Design review of the part shown in the three views and the two pictorial views. Dimensions are in mm from the part's minimum x, y and z. Coordinates: 2 decimals unless noted, no trailing zeros. Loops run counter-clockwise (first coordinate to the right, second up) from the corner with the lowest first, then second, coordinate; pieces in that order, holes last. Notation, with made-up numbers: (-33, 42) -> (6, 42) arc R21 ccw to (6, 54) -> close; hole circle Ø7 at (68.5, 56.25). An arc over 180 degrees is marked (long way). Answer in a Markdown table with one row per item.
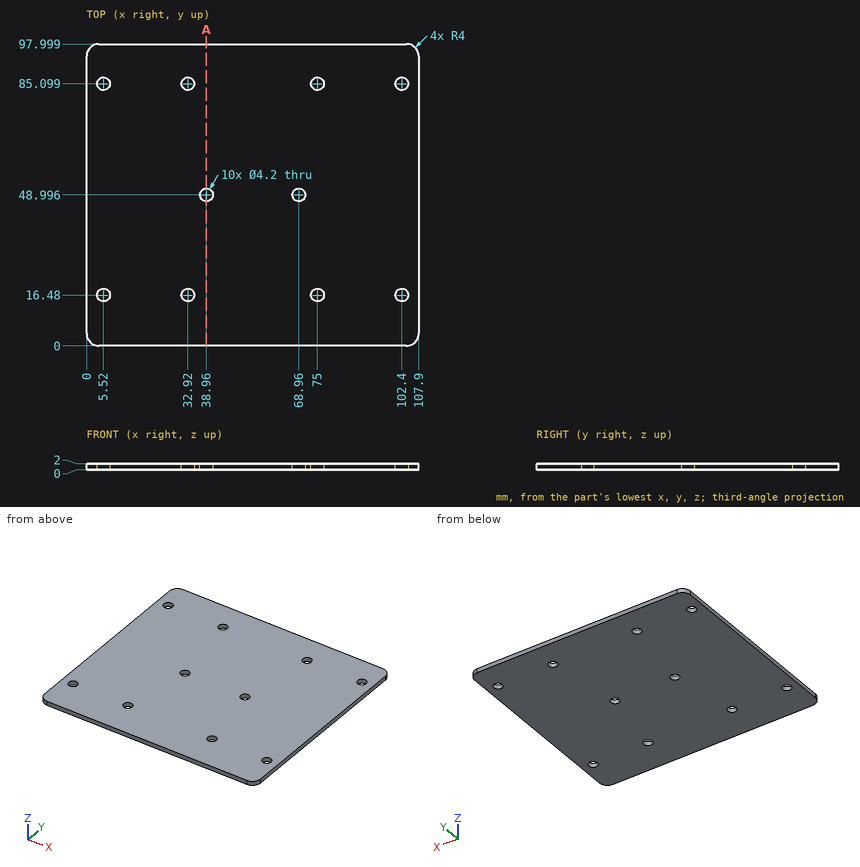
(1) For pin 1 (6.5 mm diameter, centred on x = 5.52, y = 85.1, fed in from -Z); pin 2 (4 mm diameter, centred on x = 32.92, y = 16.48, fed in from +Z), all flat-tipped, find the tip position at first contact; note any pin that passes through.
Evaluation:
| item | result |
|---|---|
| pin 1 | stops at z = 0 |
| pin 2 | passes through |
(2) To check wall thickness, follow probe 1 along Y at (x, z) = (5, 1.65) (1 decimal); probe 2 along Y at (x, z) = (69.5, 1.05) (1 decimal). State the ranges of each line that lie inside material, in increasing order.
Evaluation:
| item | result |
|---|---|
| probe 1 | y = 0 to 14.4, 18.5 to 83.1, 87.1 to 98 |
| probe 2 | y = 0 to 47, 51 to 98 |
(3) Take a section at A-A on x = 38.96. Give the boundary of the cut face in (y, z), and give its area (3 significant figures).
Evaluation:
| item | result |
|---|---|
| outline | (0, 0) -> (46.9, 0) -> (46.9, 2) -> (0, 2) -> close; (51.1, 0) -> (98, 0) -> (98, 2) -> (51.1, 2) -> close |
| area | 188 mm² |
